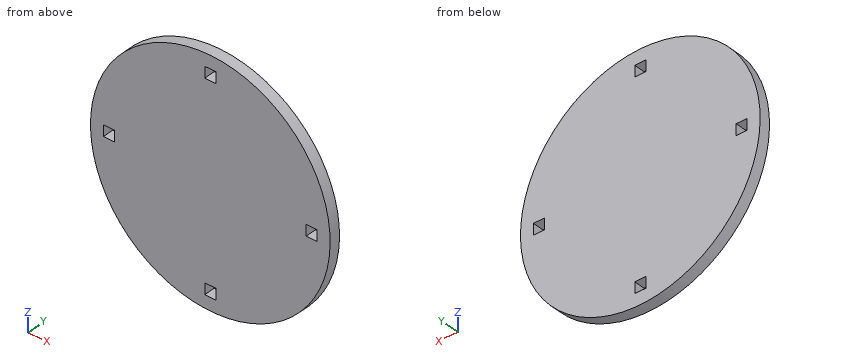
```python
from build123d import *

# Parameters (mm, degrees)
SKETCH1_R           = 32.5
BOSS_EXTRUDE1_DEPTH = 3
SKETCH3_W           = 3
SKETCH3_H           = 3
CUT_EXTRUDE4_DEPTH  = 10


with BuildPart() as part:
    # Sketch1 → Boss-Extrude1 (new body)
    with BuildSketch(Plane(origin=(0, 0, 0), x_dir=(1, 0, 0), z_dir=(0, 1, 0))):
        with Locations(Location((0, 0, 0), (0, 0, 270))):
            Circle(SKETCH1_R)
    extrude(amount=BOSS_EXTRUDE1_DEPTH)

    # Sketch3 → Cut-Extrude4 (cut)
    with BuildSketch(Plane(origin=(0, 0, 0), x_dir=(1, 0, 0), z_dir=(0, 1, 0))):
        with Locations((27.5, 0)):
            Rectangle(SKETCH3_W, SKETCH3_H)
        with Locations((0, 27.5)):
            Rectangle(SKETCH3_W, SKETCH3_H)
        with Locations((0, -27.5)):
            Rectangle(SKETCH3_W, SKETCH3_H)
        with Locations((-27.5, 0)):
            Rectangle(SKETCH3_W, SKETCH3_H)
    extrude(amount=CUT_EXTRUDE4_DEPTH, mode=Mode.SUBTRACT)


solid = part.part
```
CAD build for the part. Positions are in the model's coordinates, mm. Round coordinates to 2 decimals unless told otherwise and drop trailing zeros. Loops run counter-clockwise (first coordinate to the right, second up) from the corner with the lowest first, then second, coordinate; pieces in that order, holes last. Notation, with made-up numbers: M 25,63 L 33,63 A17 ccw 33,77 Z; hole C 84,-24 d5. An arc over 180 degrees is marked long. Return JSON: item names as keys, results as strings. Group by question number.
(1) Saw through at A-A, the plane x = 0. List the corners of the cut face in (y, z).
(2) Saw through at C-C, the plane z = 0. List the corners of the cut face in (x, y), and give its area (3 significant figures).
(3) Saw through at D-D, the plane z = 27. List the corners of the cut face in (x, y).
(4) Wall check: probe 1 along X at (y, z) = (1.2, -27); probe 2 along Z at (x, y) = (-13.5, 1.2); probe 3 along X at (y, z) = (1.55, -24.5). Give the ranges that are in metal, low to high. Write a range as [from, to].
(5) Drop flat-ended pins along their axis: P1, Ø1, axis at x = -12, y = 2, coming from the +Z side; P2, Ø1.5, axis at y = 1.5, z = 27.5, coming from the +X side; P3, Ø1, axis at x = 17, y = 2, coming from the -Z side. Give the stop position or say it passes through.
(6) Saw through at B-B, the plane y = 2.2. List the corners of the cut face in (x, z), and give its area (3 significant figures).
Answer list:
{
 "1": {"outline": "M 0,-32.5 L 3,-32.5 L 3,-29 L 0,-29 Z; M 0,-26 L 3,-26 L 3,26 L 0,26 Z; M 0,29 L 3,29 L 3,32.5 L 0,32.5 Z"},
 "2": {"outline": "M -32.5,0 L -29,0 L -29,3 L -32.5,3 Z; M -26,0 L 26,0 L 26,3 L -26,3 Z; M 29,0 L 32.5,0 L 32.5,3 L 29,3 Z", "area": "177 mm2"},
 "3": {"outline": "M -18.09,0 L -1.5,0 L -1.5,3 L -18.09,3 Z; M 1.5,0 L 18.09,0 L 18.09,3 L 1.5,3 Z"},
 "4": {"probe 1": "[-18.09, -1.5], [1.5, 18.09]", "probe 2": "[-29.56, 29.56]", "probe 3": "[-21.35, 21.35]"},
 "5": {"P1": "z = 30.4", "P2": "x = 18.46", "P3": "z = -28"},
 "6": {"outline": "C 0,0 d65; hole M -29,-1.5 L -26,-1.5 L -26,1.5 L -29,1.5 Z; hole M -1.5,-29 L 1.5,-29 L 1.5,-26 L -1.5,-26 Z; hole M -1.5,26 L 1.5,26 L 1.5,29 L -1.5,29 Z; hole M 26,-1.5 L 29,-1.5 L 29,1.5 L 26,1.5 Z", "area": "3,280 mm2"}
}
